Here's how the part is built. I have some questions about the finished solid (model axes, mm). A direction names the side the tool comes from. Coordinates: 2 decimals unless noted, no trailing zeros. Write each loop counter-clockwise with the first axis right and the second up, starting at its lowest first coordinate (ties: lowest second). Pieces come first, ordered by that corner, then holes. Notation, with made-up numbers: (26, -22) -> (34, -22) arc R32 ccw to (34, 7) -> close; hole circle Ø7 at (46, 71). An arc over 180 degrees is marked (long way). Put each result on its own line as item: value. Start each with the question number.
Item 1: On a 3-axis mill with a long thin cutter (end or side, diameter ignored), from which of +Z, -Z, +X, -X, +Y, -Y can I reach the whole of each face in a straight line? I mean faces 1 (the face through (2.77, 9.92, 2.46)), 2 (the face through (71, 5.508, 2)). Say none if no direction works.
Item 2: I want a section at D-D, the plane x = 90.5. List the corners of the cut face in (y, z) for me.
Item 3: I want a section at C-C, the plane x = 0. List the corners of the cut face in (y, z) for me.
Item 4: For pin 1 (3 mm diameter, centred on y = 7.5, z = 3.5, fed in from -X); pin 2 (1 mm diameter, centred on y = 9.5, z = 2, fed in from +X); pin 3 (3 mm diameter, centred on y = 9, z = 1.5, fed in from +X), each with a flat end and sliding along its axis, tell me the tip position at first contact or that it passes through.
Item 5: I need wall thicknesses on line 1 (X direction, y = 0.5, z = 3.85); line 2 (Y direction, x = 84, z = 0.2); line 3 (X direction, y = 4.25, z = 2.3). Which ranges of each line are inside material? Lowest first, please. Write a range as [from, to].
Item 6: I want a section at A-A, the plane z = 2.7. List the corners of the cut face in (x, y) for me, then the cut area to 3 significant figures.
Item 7: If we mould it in two halves opening along X, with no side actions, what happens to faces 3 (the face through (12.373, 16.925, 2.465)), 4 (the face through (10.48, -0.49, 2.46)), 5 (the face through (71, 9, 0))? For each: released by +X, released by -X, zero draft, split by the parting line, or undercut.
Item 8: I want a section at B-B, the plane y = 0. List the corners of the cut face in (x, z) for me.
from build123d import *

# Parameters (mm, degrees)
SCHIZZO1_R                   = 2.05
ESTRUSIONE_ESTRUSIONE1_DEPTH = 5


with BuildPart() as part:
    # Schizzo1 → Estrusione-Estrusione1 (new body)
    with BuildSketch(Plane.XY):
        with BuildLine():
            Line((-3.757019077, 4.678120099), (9.474796834, 15.30465036))
            ThreePointArc((9.474796834, 15.30465036), (12.41750963, 16.940934337), (15.736495295, 17.507783529))
            Line((15.736495295, 17.507783529), (120.577440721, 17.507783529))
            ThreePointArc((120.577440721, 17.507783529), (123.351342788, 17.115356965), (125.907534283, 15.968876995))
            Line((125.907534283, 15.968876995), (143.198056137, 5.076656079))
            ThreePointArc((143.198056137, 5.076656079), (145.076656079, -3.198056137), (136.801943863, -5.076656079))
            Line((136.801943863, -5.076656079), (122.442889956, 3.968876995))
            ThreePointArc((122.442889956, 3.968876995), (119.886698461, 5.115356965), (117.112796394, 5.507783529))
            Line((117.112796394, 5.507783529), (22.887203606, 5.507783529))
            ThreePointArc((22.887203606, 5.507783529), (20.113301539, 5.115356965), (17.557110044, 3.968876995))
            Line((17.557110044, 3.968876995), (3.198056137, -5.076656079))
            ThreePointArc((3.198056137, -5.076656079), (-4.885388875, -3.483242102), (-3.757019077, 4.678120099))
        make_face()
        Circle(SCHIZZO1_R, mode=Mode.SUBTRACT)
        with Locations((140, 0)):
            Circle(SCHIZZO1_R, mode=Mode.SUBTRACT)
    extrude(amount=ESTRUSIONE_ESTRUSIONE1_DEPTH)


solid = part.part
Calculated:
1. face 1: +Z, -Z, -X, +Y
1. face 2: +Z, -Z, -Y
2. outline: (5.51, 0) -> (17.51, 0) -> (17.51, 5) -> (5.51, 5) -> close
3. outline: (-6, 0) -> (-2.05, 0) -> (-2.05, 5) -> (-6, 5) -> close; (2.05, 0) -> (7.7, 0) -> (7.7, 5) -> (2.05, 5) -> close
4. pin 1: stops at x = -2.11
4. pin 2: stops at x = 136.97
4. pin 3: stops at x = 139.35
5. line 1: x = [-5.98, -1.99], [1.99, 12.05], [127.95, 138.01], [141.99, 145.98]
5. line 2: y = [5.51, 17.51]
5. line 3: x = [-4.24, 18.03], [121.97, 144.24]
6. outline: (-3.76, 4.68) arc R6 ccw to (3.2, -5.08) -> (17.56, 3.97) arc R10 cw to (22.89, 5.51) -> (117.11, 5.51) arc R10 cw to (122.44, 3.97) -> (136.8, -5.08) arc R6 ccw to (143.2, 5.08) -> (125.91, 15.97) arc R10 ccw to (120.58, 17.51) -> (15.74, 17.51) arc R10 ccw to (9.47, 15.3) -> close; hole circle Ø4.1 at (0, 0); hole circle Ø4.1 at (140, 0)
6. area: 1,870 mm2
7. face 3: released by -X
7. face 4: undercut
7. face 5: zero draft
8. outline: (-6, 0) -> (-2.05, 0) -> (-2.05, 5) -> (-6, 5) -> close; (2.05, 0) -> (11.26, 0) -> (11.26, 5) -> (2.05, 5) -> close; (128.74, 0) -> (137.95, 0) -> (137.95, 5) -> (128.74, 5) -> close; (142.05, 0) -> (146, 0) -> (146, 5) -> (142.05, 5) -> close
